from build123d import *

# Parameters (mm, degrees)
SKETCH4_W                = 12.46
SKETCH4_H                = 17.25
BOSS_EXTRUDE3_DEPTH      = 6
SKETCH8_R                = 12.546781182
SKETCH8_R_2              = 11.15
BOSS_EXTRUDE6_DEPTH      = 7.3
BOSS_EXTRUDE6_DEPTH_BACK = 17.25
BOSS_EXTRUDE4_DEPTH      = 17.25
SKETCH6_R                = 0.5
CUT_EXTRUDE1_DEPTH       = 20
CHAMFER1_SIZE            = 0.5
CHAMFER1_SIZE2           = 0.866025404
SKETCH10_W               = 12.46
SKETCH10_H               = 23.7
CUT_EXTRUDE3_DEPTH       = 17.25
CUT_EXTRUDE4_REACH       = 38.097
SKETCH11_W               = 5
SKETCH11_H               = 3
BOSS_EXTRUDE7_DEPTH      = 7.3
BOSS_EXTRUDE9_DEPTH      = 10
SKETCH16_R               = 11.15
SKETCH16_R_2             = 7.15
BOSS_EXTRUDE10_DEPTH     = 7.3
SKETCH17_R               = 10.15
SKETCH17_R_2             = 7.15
CUT_EXTRUDE5_DEPTH       = 1.3
SKETCH18_W               = 3
SKETCH18_H               = 10
BOSS_EXTRUDE11_DEPTH     = 5
OFFSET_R_DEPTH           = 10


with BuildPart() as part:
    # Sketch4 → Boss-Extrude3 (new body)
    with BuildSketch(Plane.XY):
        with Locations((0, -1.35)):
            Rectangle(SKETCH4_W, SKETCH4_H)
    extrude(amount=BOSS_EXTRUDE3_DEPTH)



with BuildPart() as body_2:
    # Sketch8 → Boss-Extrude6 (new body, two sides)
    with BuildSketch(Plane(origin=(0, -9.975, 0), x_dir=(-1, 0, 0), z_dir=(0, -1, 0))) as boss_extrude6_sk:
        with Locations((0, -23.55)):
            Circle(SKETCH8_R)
        with Locations((0, -23.55)):
            Circle(SKETCH8_R_2, mode=Mode.SUBTRACT)
    extrude(amount=BOSS_EXTRUDE6_DEPTH)
    extrude(boss_extrude6_sk.sketch, amount=-BOSS_EXTRUDE6_DEPTH_BACK)


with BuildPart() as part_1:
    add(part.part)

    add(body_2.part)  # Boss-Extrude4 merges body 2
    # Sketch5 → Boss-Extrude4 (add)
    with BuildSketch(Plane(origin=(0, 7.275, 0), x_dir=(1, 0, 0), z_dir=(0, 1, 0))):
        with BuildLine():
            Line((12.546781182, -23.55), (12.546781182, 0))
            Line((12.546781182, 0), (6.23, 0))
            Line((6.23, 0), (6.23, -29.7))
            Line((6.23, -29.7), (-6.23, -29.7))
            Line((-6.23, -29.7), (-6.23, 0))
            Line((-6.23, 0), (-12.546781182, 0))
            Line((-12.546781182, 0), (-12.546781182, -23.55))
            ThreePointArc((-12.546781182, -23.55), (0, -36.096781182), (12.546781182, -23.55))
        make_face()
    extrude(amount=-BOSS_EXTRUDE4_DEPTH)

    # Sketch6 → Cut-Extrude1 (cut)
    with BuildSketch(Plane(origin=(0, 7.275, 0), x_dir=(1, 0, 0), z_dir=(0, 1, 0))):
        with Locations((0, -3.6)):
            Circle(SKETCH6_R)
        with Locations((0, -32.1)):
            Circle(SKETCH6_R)
    extrude(amount=-CUT_EXTRUDE1_DEPTH, mode=Mode.SUBTRACT)

    # Chamfer1
    chamfer1_edges = [part_1.edges().sort_by_distance(p)[0] for p in [
        (-0.5, 7.275, 3.6),
        (-0.5, 7.275, 32.1),
    ]]
    chamfer1_side = [part_1.faces().sort_by_distance(p)[0] for p in [
        (0, 7.275, 35.657160381),
    ]]
    chamfer(chamfer1_edges, length=CHAMFER1_SIZE, length2=CHAMFER1_SIZE2, reference=chamfer1_side[0])

    # Sketch10 → Cut-Extrude3 (cut)
    with BuildSketch(Plane(origin=(0, 7.275, 0), x_dir=(1, 0, 0), z_dir=(0, 1, 0))):
        with Locations((0, -17.85)):
            Rectangle(SKETCH10_W, SKETCH10_H)
    extrude(amount=-CUT_EXTRUDE3_DEPTH, mode=Mode.SUBTRACT)

    # Sketch11 → Cut-Extrude4 (cut, up to next)
    with BuildSketch(Plane.XY.offset(36.096781182), mode=Mode.PRIVATE) as cut_extrude4_sk1:
        with Locations((0, -8.475)):
            Rectangle(SKETCH11_W, SKETCH11_H)
    cut_extrude4_tool1 = extrude(cut_extrude4_sk1.sketch, amount=-CUT_EXTRUDE4_REACH, mode=Mode.PRIVATE) & part_1.part
    add(cut_extrude4_tool1.solids().sort_by_distance((0, -8.475, 36.096781))[0], mode=Mode.SUBTRACT)

    # Sketch13 → Boss-Extrude7 (add)
    with BuildSketch(Plane.XZ.offset(17.275)):
        with BuildLine():
            Line((-12.546781182, 23.55), (-12.546781182, 0))
            Line((-12.546781182, 0), (12.546781182, 0))
            Line((12.546781182, 0), (12.546781182, 23.55))
            ThreePointArc((12.546781182, 23.55), (0, 11.003218818), (-12.546781182, 23.55))
        make_face()
    extrude(amount=-BOSS_EXTRUDE7_DEPTH)

    # Sketch15 → Boss-Extrude9 (add)
    with BuildSketch(Plane(origin=(0, 7.275, 0), x_dir=(1, 0, 0), z_dir=(0, 1, 0))):
        with BuildLine():
            Line((-12.546781182, 0), (12.546781182, 0))
            Line((12.546781182, 0), (12.546781182, -23.55))
            ThreePointArc((12.546781182, -23.55), (0, -36.096781182), (-12.546781182, -23.55))
            Line((-12.546781182, -23.55), (-12.546781182, 0))
        make_face()
        with BuildLine():
            Line((-6.23, -0.8), (6.23, -0.8))
            Line((6.23, -0.8), (6.23, -33.5))
            ThreePointArc((6.23, -33.5), (5.937106781, -34.207106781), (5.23, -34.5))
            Line((5.23, -34.5), (-5.23, -34.5))
            ThreePointArc((-5.23, -34.5), (-5.937106781, -34.207106781), (-6.23, -33.5))
            Line((-6.23, -33.5), (-6.23, -0.8))
        make_face(mode=Mode.SUBTRACT)
    extrude(amount=BOSS_EXTRUDE9_DEPTH)

    # Sketch16 → Boss-Extrude10 (add)
    with BuildSketch(Plane.XZ.offset(17.275)):
        with Locations((0, 23.55)):
            Circle(SKETCH16_R)
        with Locations((0, 23.55)):
            Circle(SKETCH16_R_2, mode=Mode.SUBTRACT)
    extrude(amount=-BOSS_EXTRUDE10_DEPTH)

    # Sketch17 → Cut-Extrude5 (cut)
    with BuildSketch(Plane.XZ.offset(17.275)):
        with Locations((0, 23.55)):
            Circle(SKETCH17_R)
        with Locations((0, 23.55)):
            Circle(SKETCH17_R_2, mode=Mode.SUBTRACT)
    extrude(amount=-CUT_EXTRUDE5_DEPTH, mode=Mode.SUBTRACT)

    # Sketch18 → Boss-Extrude11 (add)
    with BuildSketch(Plane.XZ.offset(17.275)):
        with Locations((8.23, 5)):
            Rectangle(SKETCH18_W, SKETCH18_H)
        with Locations((3.714, 5)):
            Rectangle(SKETCH18_W, SKETCH18_H)
    extrude(amount=BOSS_EXTRUDE11_DEPTH)

    # Sketch1 → Offset R (add)
    with BuildSketch(Plane.XY):
        Polygon((0, -75), (74.307137052, 27.275), (-74.307137052, 27.275), align=None)
    extrude(amount=-OFFSET_R_DEPTH)


solid = part_1.part
The model under review builds one solid part; all positions refer to its coordinate system, in mm. A direction names the side the tool comes from. Give positions to 0.01 mm unless a question says otherwise; leave off trailing zeros. Order: outer loops, then holes, each group sorted by start corner. A loop starts at its lowest first (then second) coordinate and runs counter-clockwise, first axis right, second up. Notation, with made-up numbers: M 22,-31 L 70,-31 A29 cw 70,-10 Z; hole C 31,79 d1. An arc over 180 degrees is marked long. Use one line per item in the form item = value. Start each with the question number.
Item 1: For faces 5 (the flat face through (4, -22.275, 5)), 6 (the cylindrical face through (-0.93, -13.02, 30.64)), 7 (the flat face through (9.73, -20, 5)), list the 3-axis set-ups (+Z, -Z, +X, -X, +Y, -Y) from which the entire face can be reached by the end or side of a thin tool; tool diameter is ignored.
Item 2: We need section B-B on z = -5. Give the boundary of the cut face in (x, y) (3 decimals), plus the area to 3 significant figures.
Item 3: We need section A-A on y = 14.5. Give the boundary of the cut face in (x, z).
Item 4: We need section D-D on y = -48. Give the boundary of the cut face in (x, z), plus the area to 3 significant figures.
Item 5: To check wall thickness, follow line 1 along Z through (x, y) = (0, -1.75); line 2 along Z through (x, y) = (0, -11.15); line 3 along X through (y, z) = (-14.25, 23.55). State the ranges of each line that lie inside material, in increasing order. Write a range as from..to.
Item 6: Insertion check: pin 1 Ø1.5 at (x, z) = (3, 6) entering from -Y (3 decimals); pin 2 Ø10 at (x, z) = (-6.5, 0.5) entering from +Y (3 decimals); pin 3 Ø1.5 at (x, z) = (-7, 12) entering from -Y (3 decimals); pin 4 Ø4 at (x, z) = (-2.5, 4) entering from +Y (3 decimals). Each pin has a flat end and moves straight along its axis. Give the tip position at first contact, or say it passes through.
Item 7: We need section C-C on x = -19.5. Give the boundary of the cut face in (y, z) (3 decimals), plus the area to 3 significant figures.
Item 8: The part is to be moulded in two halves that separate along X. For faces 1 (the flat face through (2.214, -20, 5)), 2 (the cylindrical face through (-1.321, -16.634, 33.614)), 3 (the flat face through (-7, -15.975, 21)), 4 (the flat face through (8, -20, 10)), say which applies: pulls with the +X half, pulls with the -X half, needs draft (parallel to the pull), parting line crosses it, or undercut.
Completed:
q1.face_5 = +Z, +X, -X, -Y
q1.face_6 = -Y
q1.face_7 = +Z, +X, -Y
q2.outline = M -74.307,27.275 L 0,-75 L 74.307,27.275 Z
q2.area = 7,600 mm²
q3.outline = M -65.03,-10 L 65.03,-10 L 65.03,0 L 12.55,0 L 12.55,23.55 A12.55 ccw -12.55,23.55 L -12.55,0 L -65.03,0 Z; hole M -6.23,0.8 L 6.23,0.8 L 6.23,33.5 A1 ccw 5.23,34.5 L -5.23,34.5 A1 ccw -6.23,33.5 Z
q4.outline = M -19.62,-10 L 19.62,-10 L 19.62,0 L -19.62,0 Z
q4.area = 392 mm²
q5.line_1 = -10..3.1, 4.1..6, 29.7..31.6, 32.6..36.1
q5.line_2 = -10..16.4, 30.7..36.1
q5.line_3 = -12.55..-7.15, 7.15..12.55
q6.pin_1 = -22.275
q6.pin_2 = 27.275
q6.pin_3 = -17.275
q6.pin_4 = 7.275
q7.outline = M -48.161,-10 L 27.275,-10 L 27.275,0 L -48.161,0 Z
q7.area = 754 mm²
q8.face_1 = pulls with the -X half
q8.face_2 = undercut
q8.face_3 = undercut
q8.face_4 = needs draft
